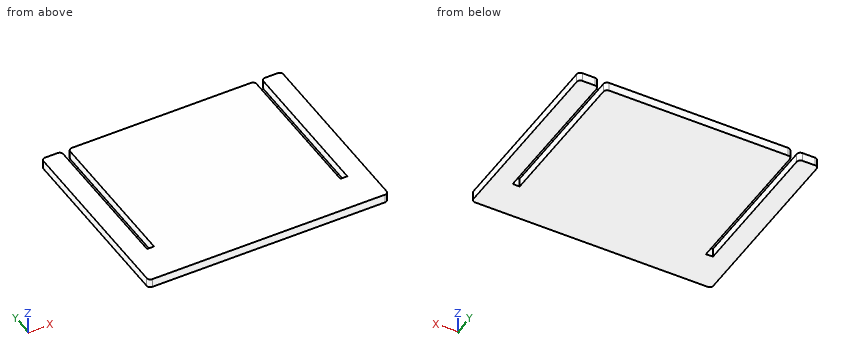
```python
from build123d import *

# Parameters (mm, degrees)
BOSS_EXTRUDE1_DEPTH = 3.175
FILLET1_R           = 1.27
SHELL1_START        = -0.1778
SHELL1_OUTLINE_W    = 80.9244
SHELL1_OUTLINE_H    = 3.5306
SHELL1_DEPTH        = 0.1778
SHELL1_START_2      = 14.942805851
SHELL1_2_OUTLINE_W  = 2.8194
SHELL1_2_OUTLINE_H  = 3.5306
SHELL1_2_DEPTH      = 0.1778
SHELL1_3_DEPTH      = 3.175
SHELL1_4_DEPTH      = 0.1778
SHELL1_START_3      = 3.175
SHELL1_5_DEPTH      = 0.1778
SHELL1_6_DEPTH      = 3.5306


with BuildPart() as part:
    # Sketch1 → Boss-Extrude1 (new body)
    with BuildSketch(Plane.XY):
        Polygon((48.26, 0), (48.26, 76.2), (10.795, 76.2), (10.795, 14.942805851), (7.62, 14.942805851), (7.62, 76.2), (0, 76.2), (0, 0), align=None)
        Polygon((85.725, 76.2), (48.26, 76.2), (48.26, 0), (96.52, 0), (96.52, 76.2), (88.9, 76.2), (88.9, 14.942805851), (85.725, 14.942805851), align=None)
    extrude(amount=BOSS_EXTRUDE1_DEPTH)

    # Fillet1
    fillet1_edges = [part.edges().sort_by_distance(p)[0] for p in [
        (0, 0, 1.5875),
        (0, 76.2, 1.5875),
        (7.62, 76.2, 1.5875),
        (10.795, 76.2, 1.5875),
        (85.725, 76.2, 1.5875),
        (88.9, 76.2, 1.5875),
        (96.52, 76.2, 1.5875),
        (96.52, 0, 1.5875),
    ]]
    fillet(fillet1_edges, radius=FILLET1_R)

    # Shell1: read off the stored shape, not the designer's step
    # Shell1 outline → Shell1 (add)
    with BuildSketch(Plane(origin=(0, 0, 0), x_dir=(1, 0, 0), z_dir=(0, 1, 0)).offset(SHELL1_START)):
        with Locations((48.26, -1.5875)):
            Rectangle(SHELL1_OUTLINE_W, SHELL1_OUTLINE_H)
    extrude(amount=SHELL1_DEPTH)

    # Shell1 2 outline → Shell1 2 (add)
    with BuildSketch(Plane(origin=(0, 0, 0), x_dir=(1, 0, 0), z_dir=(0, 1, 0)).offset(SHELL1_START_2)):
        with Locations((87.3125, -1.5875)):
            Rectangle(SHELL1_2_OUTLINE_W, SHELL1_2_OUTLINE_H)
        with Locations((9.2075, -1.5875)):
            Rectangle(SHELL1_2_OUTLINE_W, SHELL1_2_OUTLINE_H)
    extrude(amount=SHELL1_2_DEPTH)

    # Shell1 3 outline → Shell1 3 (cut)
    with BuildSketch(Plane.XY):
        with BuildLine():
            Line((1.27, 0), (95.25, 0))
            ThreePointArc((95.25, 0), (96.148025612, 0.371974388), (96.52, 1.27))
            Line((96.52, 1.27), (96.52, 74.93))
            ThreePointArc((96.52, 74.93), (96.148025612, 75.828025612), (95.25, 76.2))
            Line((95.25, 76.2), (90.17, 76.2))
            ThreePointArc((90.17, 76.2), (89.271974388, 75.828025612), (88.9, 74.93))
            Line((88.9, 74.93), (88.9, 14.942805851))
            Line((88.9, 14.942805851), (85.725, 14.942805851))
            Line((85.725, 14.942805851), (85.725, 74.93))
            ThreePointArc((85.725, 74.93), (85.353025612, 75.828025612), (84.455, 76.2))
            Line((84.455, 76.2), (12.065, 76.2))
            ThreePointArc((12.065, 76.2), (11.166974388, 75.828025612), (10.795, 74.93))
            Line((10.795, 74.93), (10.795, 14.942805851))
            Line((10.795, 14.942805851), (7.62, 14.942805851))
            Line((7.62, 14.942805851), (7.62, 74.93))
            ThreePointArc((7.62, 74.93), (7.248025612, 75.828025612), (6.35, 76.2))
            Line((6.35, 76.2), (1.27, 76.2))
            ThreePointArc((1.27, 76.2), (0.371974388, 75.828025612), (0, 74.93))
            Line((0, 74.93), (0, 1.27))
            ThreePointArc((0, 1.27), (0.371974388, 0.371974388), (1.27, 0))
        make_face()
    extrude(amount=SHELL1_3_DEPTH, mode=Mode.SUBTRACT)

    # Shell1 4 outline → Shell1 4 (add)
    with BuildSketch(Plane.XY.offset(SHELL1_START)):
        with BuildLine():
            Line((96.6978, 1.27), (96.6978, 74.93))
            ThreePointArc((96.6978, 74.93), (96.273749198, 75.953749198), (95.25, 76.3778))
            Line((95.25, 76.3778), (90.17, 76.3778))
            ThreePointArc((90.17, 76.3778), (89.146250802, 75.953749198), (88.7222, 74.93))
            Line((88.7222, 74.93), (88.7222, 14.942805851))
            Line((88.7222, 14.942805851), (85.9028, 14.942805851))
            Line((85.9028, 14.942805851), (85.9028, 74.93))
            ThreePointArc((85.9028, 74.93), (85.478749198, 75.953749198), (84.455, 76.3778))
            Line((84.455, 76.3778), (12.065, 76.3778))
            ThreePointArc((12.065, 76.3778), (11.041250802, 75.953749198), (10.6172, 74.93))
            Line((10.6172, 74.93), (10.6172, 14.942805851))
            Line((10.6172, 14.942805851), (7.7978, 14.942805851))
            Line((7.7978, 14.942805851), (7.7978, 74.93))
            ThreePointArc((7.7978, 74.93), (7.373749198, 75.953749198), (6.35, 76.3778))
            Line((6.35, 76.3778), (1.27, 76.3778))
            ThreePointArc((1.27, 76.3778), (0.246250802, 75.953749198), (-0.1778, 74.93))
            Line((-0.1778, 74.93), (-0.1778, 1.27))
            ThreePointArc((-0.1778, 1.27), (0.246250802, 0.246250802), (1.27, -0.1778))
            Line((1.27, -0.1778), (7.7978, -0.1778))
            Line((7.7978, -0.1778), (7.7978, 0))
            Line((7.7978, 0), (88.7222, 0))
            Line((88.7222, 0), (88.7222, -0.1778))
            Line((88.7222, -0.1778), (95.25, -0.1778))
            ThreePointArc((95.25, -0.1778), (96.273749198, 0.246250802), (96.6978, 1.27))
        make_face()
    extrude(amount=SHELL1_4_DEPTH)

    # Shell1 5 outline → Shell1 5 (add)
    with BuildSketch(Plane.XY.offset(SHELL1_START_3)):
        with BuildLine():
            Line((96.6978, 1.27), (96.6978, 74.93))
            ThreePointArc((96.6978, 74.93), (96.273749198, 75.953749198), (95.25, 76.3778))
            Line((95.25, 76.3778), (90.17, 76.3778))
            ThreePointArc((90.17, 76.3778), (89.146250802, 75.953749198), (88.7222, 74.93))
            Line((88.7222, 74.93), (88.7222, 14.942805851))
            Line((88.7222, 14.942805851), (85.9028, 14.942805851))
            Line((85.9028, 14.942805851), (85.9028, 74.93))
            ThreePointArc((85.9028, 74.93), (85.478749198, 75.953749198), (84.455, 76.3778))
            Line((84.455, 76.3778), (12.065, 76.3778))
            ThreePointArc((12.065, 76.3778), (11.041250802, 75.953749198), (10.6172, 74.93))
            Line((10.6172, 74.93), (10.6172, 14.942805851))
            Line((10.6172, 14.942805851), (7.7978, 14.942805851))
            Line((7.7978, 14.942805851), (7.7978, 74.93))
            ThreePointArc((7.7978, 74.93), (7.373749198, 75.953749198), (6.35, 76.3778))
            Line((6.35, 76.3778), (1.27, 76.3778))
            ThreePointArc((1.27, 76.3778), (0.246250802, 75.953749198), (-0.1778, 74.93))
            Line((-0.1778, 74.93), (-0.1778, 1.27))
            ThreePointArc((-0.1778, 1.27), (0.246250802, 0.246250802), (1.27, -0.1778))
            Line((1.27, -0.1778), (7.7978, -0.1778))
            Line((7.7978, -0.1778), (7.7978, 0))
            Line((7.7978, 0), (88.7222, 0))
            Line((88.7222, 0), (88.7222, -0.1778))
            Line((88.7222, -0.1778), (95.25, -0.1778))
            ThreePointArc((95.25, -0.1778), (96.273749198, 0.246250802), (96.6978, 1.27))
        make_face()
    extrude(amount=SHELL1_5_DEPTH)

    # Shell1 6 outline → Shell1 6 (add)
    with BuildSketch(Plane.XY.offset(SHELL1_START)):
        with BuildLine():
            Line((96.6978, 1.27), (96.6978, 74.93))
            ThreePointArc((96.6978, 74.93), (96.273749198, 75.953749198), (95.25, 76.3778))
            Line((95.25, 76.3778), (90.17, 76.3778))
            ThreePointArc((90.17, 76.3778), (89.146250802, 75.953749198), (88.7222, 74.93))
            Line((88.7222, 74.93), (88.7222, 14.942805851))
            Line((88.7222, 14.942805851), (88.9, 14.942805851))
            Line((88.9, 14.942805851), (88.9, 74.93))
            ThreePointArc((88.9, 74.93), (89.271974388, 75.828025612), (90.17, 76.2))
            Line((90.17, 76.2), (95.25, 76.2))
            ThreePointArc((95.25, 76.2), (96.148025612, 75.828025612), (96.52, 74.93))
            Line((96.52, 74.93), (96.52, 1.27))
            ThreePointArc((96.52, 1.27), (96.148025612, 0.371974388), (95.25, 0))
            Line((95.25, 0), (88.7222, 0))
            Line((88.7222, 0), (88.7222, -0.1778))
            Line((88.7222, -0.1778), (95.25, -0.1778))
            ThreePointArc((95.25, -0.1778), (96.273749198, 0.246250802), (96.6978, 1.27))
        make_face()
        with BuildLine():
            Line((1.27, -0.1778), (7.7978, -0.1778))
            Line((7.7978, -0.1778), (7.7978, 0))
            Line((7.7978, 0), (1.27, 0))
            ThreePointArc((1.27, 0), (0.371974388, 0.371974388), (0, 1.27))
            Line((0, 1.27), (0, 74.93))
            ThreePointArc((0, 74.93), (0.371974388, 75.828025612), (1.27, 76.2))
            Line((1.27, 76.2), (6.35, 76.2))
            ThreePointArc((6.35, 76.2), (7.248025612, 75.828025612), (7.62, 74.93))
            Line((7.62, 74.93), (7.62, 14.942805851))
            Line((7.62, 14.942805851), (7.7978, 14.942805851))
            Line((7.7978, 14.942805851), (7.7978, 74.93))
            ThreePointArc((7.7978, 74.93), (7.373749198, 75.953749198), (6.35, 76.3778))
            Line((6.35, 76.3778), (1.27, 76.3778))
            ThreePointArc((1.27, 76.3778), (0.246250802, 75.953749198), (-0.1778, 74.93))
            Line((-0.1778, 74.93), (-0.1778, 1.27))
            ThreePointArc((-0.1778, 1.27), (0.246250802, 0.246250802), (1.27, -0.1778))
        make_face()
        with BuildLine():
            Line((85.725, 14.942805851), (85.9028, 14.942805851))
            Line((85.9028, 14.942805851), (85.9028, 74.93))
            ThreePointArc((85.9028, 74.93), (85.478749198, 75.953749198), (84.455, 76.3778))
            Line((84.455, 76.3778), (12.065, 76.3778))
            ThreePointArc((12.065, 76.3778), (11.041250802, 75.953749198), (10.6172, 74.93))
            Line((10.6172, 74.93), (10.6172, 14.942805851))
            Line((10.6172, 14.942805851), (10.795, 14.942805851))
            Line((10.795, 14.942805851), (10.795, 74.93))
            ThreePointArc((10.795, 74.93), (11.166974388, 75.828025612), (12.065, 76.2))
            Line((12.065, 76.2), (84.455, 76.2))
            ThreePointArc((84.455, 76.2), (85.353025612, 75.828025612), (85.725, 74.93))
            Line((85.725, 74.93), (85.725, 14.942805851))
        make_face()
    extrude(amount=SHELL1_6_DEPTH)


solid = part.part
```
Build history of the part. All positions in model axes, mm. Round coordinates to 2 decimals unless told otherwise and drop trailing zeros. Write each loop counter-clockwise with the first axis right and the second up, starting at its lowest first coordinate (ties: lowest second). Pieces come first, ordered by that corner, then holes.
1) Band-saw the part on A-A, the plane y = 33.5. List the corners of the cut face in (x, z) (3 decimals), and give its area (3 significant figures).
2) Band-saw the part on C-C, the plane y = 11. List the corners of the cut face in (x, z) (3 decimals), and give its area (3 significant figures).
3) Drill centre lines: probe 1 along X at (y, z) = (42, 1.9) (3 decimals); probe 2 along Y at (x, z) = (88, 1.4); probe 3 along X at (y, z) = (10.5, 2.45). Where is each one in solid material? Low to high.
4) Band-saw the part on B-B, the plane x = 29.5. List the corners of the cut face in (y, z) (3 decimals).
Ans:
1. outline: (-0.178, -0.178) - (7.798, -0.178) - (7.798, 3.353) - (-0.178, 3.353) - close; (10.617, -0.178) - (85.903, -0.178) - (85.903, 3.353) - (10.617, 3.353) - close; (88.722, -0.178) - (96.698, -0.178) - (96.698, 3.353) - (88.722, 3.353) - close; hole (0, 0) - (7.62, 0) - (7.62, 3.175) - (0, 3.175) - close; hole (10.795, 0) - (85.725, 0) - (85.725, 3.175) - (10.795, 3.175) - close; hole (88.9, 0) - (96.52, 0) - (96.52, 3.175) - (88.9, 3.175) - close
1. area: 35.8 mm2
2. outline: (-0.178, -0.178) - (96.698, -0.178) - (96.698, 3.353) - (-0.178, 3.353) - close; hole (0, 0) - (96.52, 0) - (96.52, 3.175) - (0, 3.175) - close
2. area: 35.6 mm2
3. probe 1: x = -0.178 to 0, 7.62 to 7.798, 10.617 to 10.795, 85.725 to 85.903, 88.722 to 88.9, 96.52 to 96.698
3. probe 2: y = -0.18 to 0, 14.94 to 15.12
3. probe 3: x = -0.18 to 0, 96.52 to 96.7
4. outline: (-0.178, -0.178) - (76.378, -0.178) - (76.378, 3.353) - (-0.178, 3.353) - close; hole (0, 0) - (76.2, 0) - (76.2, 3.175) - (0, 3.175) - close
